The model under review builds one solid part; all positions refer to its coordinate system, in mm. A direction names the side the tool comes from. Coordinates: 2 decimals unless noted, no trailing zeros. Write each loop counter-clockwise with the first axis right and the second up, starting at its lowest first coordinate (ties: lowest second). Pieces come first, ordered by that corner, then holes. Notation, with made-up numbers: (-5, 59.5) - (45, 59.5) arc R31 ccw to (45, 95.5) - close; hole circle Ø4 at (74, 0). An arc over 180 degrees is marked (long way). Return JSON: item names as keys, results as strings. Group by question number.
(1) We need section C-C on x = -17. State the section outline as (y, z) points, then the cut area to 3 significant figures.
(2) Tool access review of faces 5 (the face through (-25.58, 25.655, 16.258)), 6 (the face through (-8, -1, 0)), 7 (the face through (0, 0, 10)): name each direction out of +Z, -Z, +X, -X, +Y, -Y from which nothing blocks a thin tool from reaching the whole face with its end or side.
(3) To check wall thickness, follow L1, parallel to X at y = 0, z = 8; L2, parallel to Z at x = 13.5, y = -29.5; L3, parallel to Z at x = -4.5, y = 3. State the ranges of each line that lie inside material, in increasing order. Write a range as from..to.
(4) For pin 1 Ø2 at (x, y) = (-24.75, -24.75) entering from +Z; pin 2 Ø6 at (y, z) = (27, 22) entering from +X; pin 3 Ø4 at (x, y) = (0, 15.75) entering from +Z, all flat-tipped, find the tip position at first contact; note any pin that passes through.
(5) Draft analysis for pull direction X (two halves, no side actions). For faces 1 (the face through (-4.336, 19.524, 22.504)), 2 (the face through (9.4, -18.3, 19.3)), 3 (the face through (-2.17, -9.76, 23.83)), 4 (the face through (11.44, 10.944, 16.774)), state which applies: released by +X, released by -X, zero draft, split by the parting line, or undercut.
(6) We need section A-A on y = 0. State the section outline as (x, z) points.
(7) We need section B-B on z = 3. State the section outline as (x, y) points.
(8) We need section D-D on x = 32. State the section outline as (y, z) points.
Autodesk Inventor part; units mm, degrees
ref_plane "YZ Plane" through (0, 0, 0) normal (1, 0, 0) x (0, 1, 0)
ref_plane "XZ Plane" through (0, 0, 0) normal (0, 1, 0) x (-1, 0, 0)
ref_plane "XY Plane" through (0, 0, 0) normal (0, 0, 1) x (1, 0, 0)
sketch "スケッチ1" plane through (0, 0, 0) normal (0, 1, 0) x (-1, 0, 0)
  circle A0 centre (0, 0) radius 40
  dimension "d0" = 80
extrude "押し出し1" add sketch "スケッチ1" along normal blind 19.3
sketch "スケッチ3" plane through (0, 19.3, 0) normal (0, 1, 0) x (1, 0, 0)
  circle A0 centre (0, 0) radius 20
  dimension "d3" = 40
extrude "押し出し2" add sketch "スケッチ3" along normal blind 6.5
sketch "スケッチ4" plane through (0, 25.8, 0) normal (0, 1, 0) x (1, 0, 0)
  circle A0 centre (0, 0) radius 10
  dimension "d6" = 20
extrude "押し出し3" cut sketch "スケッチ4" against normal blind 4
sketch "スケッチ5" plane through (0, 19.3, 0) normal (0, 1, 0) x (1, 0, 0)
  point P0 (0, 0)
  point P1 (0, 0)
  point P2 (-24.7487, -24.7487)
  point P3 (24.7487, -24.7487)
  point P4 (24.7487, 24.7487)
  point P5 (-24.7487, 24.7487)
  dimension "d9" = 35
  dimension "d12" = 360
hole "穴1" at (-24.7487, 19.3, -24.7487) at (-24.7487, 19.3, 24.7487) at (24.7487, 19.3, 24.7487) at (24.7487, 19.3, -24.7487) direction (0, -1, 0) diameter 2.459 depth 6 tip angle 118
sketch "スケッチ6" plane through (0, 25.8, 0) normal (0, 1, 0) x (1, 0, 0)
  point P0 (0, 0)
  point P1 (-11.1369, -11.1369)
  point P2 (11.1369, -11.1369)
  point P3 (11.1369, 11.1369)
  point P4 (-11.1369, 11.1369)
  dimension "d21" = 15.75
  dimension "d24" = 360
hole "穴2" at (-11.1369, 25.8, 11.1369) at (11.1369, 25.8, 11.1369) at (11.1369, 25.8, -11.1369) at (-11.1369, 25.8, -11.1369) direction (0, -1, 0) diameter 4.134 depth 8 tip angle 118
sketch "スケッチ7" plane through (0, 25.8, 0) normal (0, 1, 0) x (1, 0, 0)
  point P0 (0, 0)
  point P1 (0, 15.75)
  dimension "d33" = 15.75
hole "穴3" at (0, 25.8, -15.75) direction (0, -1, 0) diameter 5 depth 8 tip angle 118
sketch "スケッチ8" plane through (0, 0, 0) normal (0, -1, 0) x (1, 0, 0)
  circle A0 centre (0, 0) radius 5
  dimension "d41" = 10
extrude "押し出し4" cut sketch "スケッチ8" against normal blind 10
move or copy body "ボディを移動2" bodies to move or copy 1 copy no rotation origin (0, 0, 0) rotation axis (1, 0, 0) rotation angle 90
properties part number "HandMountingFlange" material "PAEK 樹脂"
Ans:
{
 "1": {"outline": "(-36.21, 0) - (36.21, 0) - (36.21, 19.3) - (10.54, 19.3) - (10.54, 25.8) - (-10.54, 25.8) - (-10.54, 19.3) - (-36.21, 19.3) - close", "area": "1,530 mm²"},
 "2": {"face 5": "+Z", "face 6": "-Z, +X, -X, +Y, -Y", "face 7": "-Z"},
 "3": {"L1": "-40..-5, 5..40", "L2": "0..19.3", "L3": "0..21.8"},
 "4": {"pin 1": "z = 13.16", "pin 2": "x = 30.66", "pin 3": "z = 17.5"},
 "5": {"face 1": "split by the parting line", "face 2": "zero draft", "face 3": "undercut", "face 4": "undercut"},
 "6": {"outline": "(-40, 0) - (-5, 0) - (-5, 10) - (5, 10) - (5, 0) - (40, 0) - (40, 19.3) - (20, 19.3) - (20, 25.8) - (10, 25.8) - (10, 21.8) - (-10, 21.8) - (-10, 25.8) - (-20, 25.8) - (-20, 19.3) - (-40, 19.3) - close"},
 "7": {"outline": "circle Ø80 at (0, 0); hole circle Ø10 at (0, 0)"},
 "8": {"outline": "(-24, 0) - (24, 0) - (24, 19.3) - (-24, 19.3) - close"}
}
